```python
from build123d import *

# Parameters (mm, degrees)
F0_W          = 25.4
F0_H          = 25.4
F1_DEPTH      = 2.54
F2_R          = 6.3627
F3_DEPTH      = 25.4
F3_DEPTH_BACK = 25.4
F4_W          = 25.3639966249
F4_H          = 3.2993815839
F5_DEPTH      = 25.4
F6_R          = 2.4136408641
F7_DEPTH      = 52.07


with BuildPart() as f1:
    # F0 (on Top) → F1 (new body)
    with BuildSketch(Plane.XY):
        with Locations((12.7, -12.7)):
            Rectangle(F0_W, F0_H)
    extrude(amount=F1_DEPTH)

    # F2 (on Top) → F3 (cut, two sides)
    with BuildSketch(Plane.XY) as f3_sk:
        with Locations((12.7851041034, -8.867087774)):
            Circle(F2_R)
    extrude(amount=-F3_DEPTH, mode=Mode.SUBTRACT)
    extrude(f3_sk.sketch, amount=F3_DEPTH_BACK, mode=Mode.SUBTRACT)

    # F4 (on Top) → F5 (join)
    with BuildSketch(Plane.XY):
        with Locations((12.6819983125, -23.7143039703)):
            Rectangle(F4_W, F4_H)
    extrude(amount=F5_DEPTH)

    # F6 (on Front) → F7 (cut)
    with BuildSketch(Plane.XZ):
        with Locations((22.2708247602, 14.8472161964)):
            Circle(F6_R)
        with Locations((3.1737023965, 14.8472161964)):
            Circle(F6_R)
    extrude(amount=F7_DEPTH, mode=Mode.SUBTRACT)


solid = f1.part
```
Check sheet for the modelled part. Datum: model origin and axes. Units: mm. A direction names the side the tool comes from. Round coordinates to 2 decimals unless told otherwise and drop trailing zeros. Order: outer loops, then holes, each group sorted by start corner. A loop starts at its lowest first (then second) coordinate and runs counter-clockwise, first axis right, second up. Notation, with made-up numbers: M 23,73.5 L 62,73.5 A14 cw 62,97.5 Z; hole C -39.5,43.25 d10. An arc over 180 degrees is marked long. Answer in a Markdown table with one row per item.
(1) Section check B-B on z = 13.5. Record the boundary of the cut face in (x, y).
Findings:
| item | result |
|---|---|
| outline | M 0,-25.36 L 1.17,-25.36 L 1.17,-22.06 L 0,-22.06 Z; M 5.18,-25.36 L 20.27,-25.36 L 20.27,-22.06 L 5.18,-22.06 Z; M 24.27,-25.36 L 25.36,-25.36 L 25.36,-22.06 L 24.27,-22.06 Z |
(2) Section check C-C on y = -12.75. Record the boundary of the cut face in (x, z), plus the area to 3 significant figures.
Findings:
| item | result |
|---|---|
| outline | M 0,0 L 7.74,0 L 7.74,2.54 L 0,2.54 Z; M 17.83,0 L 25.4,0 L 25.4,2.54 L 17.83,2.54 Z |
| area | 38.9 mm^2 |
(3) Section check D-D on y = -23. Give the number of separate pieces and of enclosed holes in the cut face, plus the area to 3 significant figures.
Findings:
| item | result |
|---|---|
| separate pieces | 1 |
| enclosed holes | 2 |
| area | 608 mm^2 |
(4) Set-up check for faces 4 (the flat face through (13, -25.364, 14)), 5 (the flat face through (25.364, -24, 14)), 6 (the flat face through (13, -24, 25.4)): record each of +Z, -Z, +X, -X, +Y, -Y from which the full face is reachable in a straight line by a thin tool's end or side.
Findings:
| item | result |
|---|---|
| face 4 | +Z, +X, -X, -Y |
| face 5 | +Z, +X, +Y, -Y |
| face 6 | +Z, +X, -X, +Y, -Y |
(5) Gauge pin test, flat ends, axial feed: pin 1 (11.5 mm diameter, centred on x = 16.5, z = 19.5, fed in from +Y); pin 2 (11.5 mm diameter, centred on x = 9, z = 11.5, fed in from -Y); pin 3 (1.6 mm diameter, centred on y = -23, z = 8.5, fed in from +X). Record the tip position at first contact, or that the pin passes through.
Findings:
| item | result |
|---|---|
| pin 1 | stops at y = -22.06 |
| pin 2 | stops at y = -25.36 |
| pin 3 | stops at x = 25.36 |
(6) Material ranges on line 1 along Y through (x, z) = (10.75, 23.75); line 2 along Z through (x, y) = (18.75, -4); line 3 along X through (y, z) = (-22.75, 6.5), recorded low to high. Write a range as from..to.
Findings:
| item | result |
|---|---|
| line 1 | y = -25.36..-22.06 |
| line 2 | z = 0..2.54 |
| line 3 | x = 0..25.36 |
(7) Draft check along X on faces 1 (the flat face through (13, -22.065, 14)), 2 (the flat face through (25.4, -13, 1)), 3 (the cylindrical face through (24.573, -23.691, 15.572)). Enter one of: +X half, -X half, draft (parallel to the pull), parting line (faces both ways), or undercut.
Findings:
| item | result |
|---|---|
| face 1 | draft |
| face 2 | +X half |
| face 3 | undercut |
